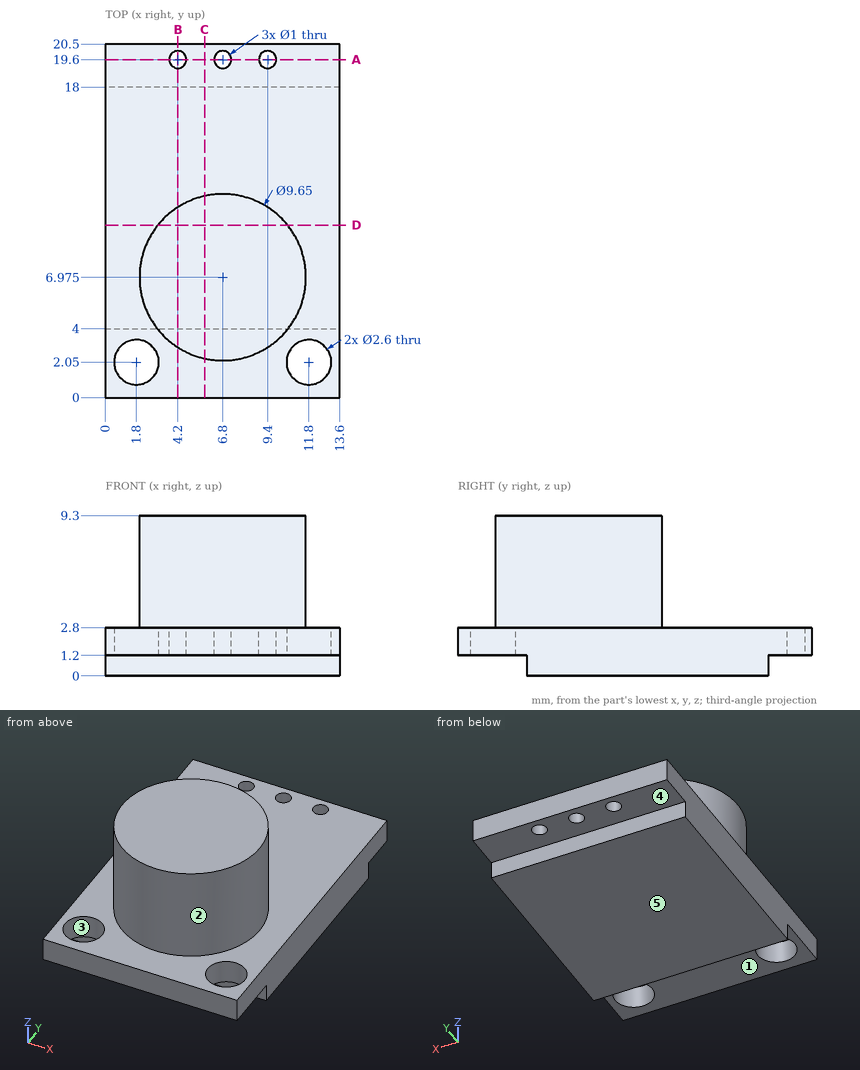
Input: dimensioned drawing with shaded views. Units: mm. Origin: part minimum x, y, z. A direction names the side the tool comes from. Round coordinates to 2 decimals unless told otherwise and drop trailing zeros. Write each loop counter-clockwise with the first axis right and the second up, starting at its lowest first coordinate (ties: lowest second). Pieces come first, ordered by that corner, then holes. Notation, with made-up numbers: (50, 40) - (103, 40) arc R32 cw to (103, 69) - close; hole circle Ø6 at (15.5, 67.5). An arc over 180 degrees is marked (long way). Write item = value, one per line.
(1) Access query for the marked faces 4 and 5. Directions: +Z, -Z, +X, -X, +Y, -Y. A direction counts if a zero-diameter tool reaches every point of the face in a straight line with its end or side. Return the directions, or none.
Geometry check:
face_4 = -Z, +X, -X, +Y
face_5 = -Z, +X, -X, +Y, -Y
(2) Material intervals for probe 1 along X at (y, z) = (19.6, 2.35); probe 2 along X at (y, z) = (2.05, 1.8); probe 3 along Y at (x, z) = (6.8, 2.05), sorted ascending.
Geometry check:
probe_1 = 0 to 3.7, 4.7 to 6.3, 7.3 to 8.9, 9.9 to 13.6
probe_2 = 0 to 0.5, 3.1 to 10.5, 13.1 to 13.6
probe_3 = 0 to 19.1, 20.1 to 20.5
(3) Pull-direction query (X, two-part tool) for the marked faces 1, 2 and 3; classes: +X half, -X half, draft (parallel to the pull), parting line (faces both ways), or undercut.
Geometry check:
face_1 = draft
face_2 = parting line
face_3 = undercut
(4) Section query D-D on y = 10. Output: boundary loops of the cut face in (x, z).
Geometry check:
outline = (0, 0) - (13.6, 0) - (13.6, 2.8) - (10.56, 2.8) - (10.56, 9.3) - (3.04, 9.3) - (3.04, 2.8) - (0, 2.8) - close
(5) Section query C-C on x = 5.75. Output: boundary loops of the cut face in (y, z).
Geometry check:
outline = (0, 1.2) - (4, 1.2) - (4, 0) - (18, 0) - (18, 1.2) - (20.5, 1.2) - (20.5, 2.8) - (11.68, 2.8) - (11.68, 9.3) - (2.27, 9.3) - (2.27, 2.8) - (0, 2.8) - close
(6) Section query B-B on x = 4.2. Output: boundary loops of the cut face in (y, z).
Geometry check:
outline = (0, 1.2) - (4, 1.2) - (4, 0) - (18, 0) - (18, 1.2) - (19.1, 1.2) - (19.1, 2.8) - (11.04, 2.8) - (11.04, 9.3) - (2.91, 9.3) - (2.91, 2.8) - (0, 2.8) - close; (20.1, 1.2) - (20.5, 1.2) - (20.5, 2.8) - (20.1, 2.8) - close
(7) Section query A-A on y = 19.6. Output: boundary loops of the cut face in (x, z).
Geometry check:
outline = (0, 1.2) - (3.7, 1.2) - (3.7, 2.8) - (0, 2.8) - close; (4.7, 1.2) - (6.3, 1.2) - (6.3, 2.8) - (4.7, 2.8) - close; (7.3, 1.2) - (8.9, 1.2) - (8.9, 2.8) - (7.3, 2.8) - close; (9.9, 1.2) - (13.6, 1.2) - (13.6, 2.8) - (9.9, 2.8) - close
(8) Contact query for flat-ended pins moving along their axis: pin 1 Ø1 at (x, z) = (10, 0.5) entering from -Y; pin 2 Ø3.5 at (x, y) = (11.8, 2.05) entering from -Z; pin 3 Ø2 at (y, z) = (17.5, 4) entering from -X; pin 4 Ø2 at (x, y) = (1.5, 10.5) entering from +Z. Output: stop coordinate, or through.
Geometry check:
pin_1 = 4
pin_2 = 1.2
pin_3 = through
pin_4 = 2.8
